The model under review builds one solid part; all positions refer to its coordinate system, in mm. Face numbers are marked on the shaded views. A direction names the side the tool comes from. Round coordinates to 2 decimals unless told otherwise and drop trailing zeros. Loops run counter-clockwise (first coordinate to the right, second up) from the corner with the lowest first, then second, coordinate; pieces in that order, holes last. Notation, with made-up numbers: (73, 62) -> (79, 62) arc R30 cw to (79, 101) -> close; hole circle Ø2 at (41, -18.75). An arc over 180 degrees is marked (long way). Write each question's results on one line, items separated by ' | '. Start each with the question number.
Item 1: Mouldability with a two-part tool opening along X and no side actions: class the marked faces 1, 2, 3 and 4 as pulls with the +X half, pulls with the -X half, needs draft (parallel to the pull), parting line crosses it, or undercut.
Item 2: Clearance check with flat-ended pins moving along their axes: pin 1 Ø2.5 at (y, z) = (0, 3) entering from -X; pin 2 Ø3.5 at (y, z) = (0, 3) entering from -X; pin 3 Ø2 at (x, z) = (-5.5, 4) entering from -Y; pin 4 Ø2 at (x, z) = (-7.5, 2) entering from -Y. State where each tip first meets the part, or that it passes through.
Item 3: We need section A-A (y = 0). Give the boundary of the cut face in (x, z).
Item 4: For L1, parallel to Z at x = -11.8, y = 0; L2, parallel to X at y = 6.5, z = 4.8; L3, parallel to Y at x = 0, z = 5.45, list the stretches that pass through material, from the lowest coordinate up. Write a range as from..to.
Item 5: Tool access review of the marked faces 5, 6 and 7: name each direction out of +Z, -Z, +X, -X, +Y, -Y from which nothing blocks a thin tool from reaching the whole face with its end or side.
Item 6: We need section C-C (x = 5). Give the boundary of the cut face in (y, z).
Item 7: We need section B-B (z = 0.4). Give the boundary of the cut face in (x, y).
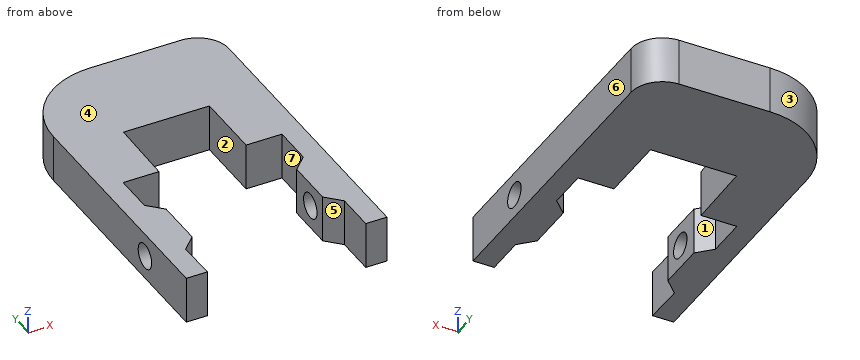
from build123d import *

# Parameters (mm, degrees)
PAD016_DEPTH    = 6
FILLET003_R     = 4
FILLET004_R     = 10
SKETCH047_R     = 1.6
POCKET022_DEPTH = 40


with BuildPart() as part:
    # Sketch046 → Pad016 (new body)
    with BuildSketch(Plane.XY):
        Polygon((10.115871, -9.866412), (10.115871, -4.766412), (8.315871, -2.966412), (8.315871, 3.233588), (10.115871, 5.033588), (10.115871, 10.133588), (5.545871, 10.133588), (5.545871, 18.880948), (-5.414129, 18.879181), (-5.564129, 10.133108), (-10.134129, 10.133108), (-10.134129, 5.033108), (-8.334129, 3.233108), (-8.334129, -2.966892), (-10.134129, -4.766892), (-10.064129, -9.866412), (-12.770461, -9.866412), (-12.770461, 31.817863), (12.822202, 31.817863), (12.822202, -9.866412), align=None)
    extrude(amount=PAD016_DEPTH)

    # Fillet003
    fillet003_edges = [part.edges().sort_by_distance(p)[0] for p in [
        (12.822202, 31.817863, 3),
    ]]
    fillet(fillet003_edges, radius=FILLET003_R)

    # Fillet004
    fillet004_edges = [part.edges().sort_by_distance(p)[0] for p in [
        (-12.770461, 31.817863, 3),
    ]]
    fillet(fillet004_edges, radius=FILLET004_R)

    # Sketch047 (on Face6 of Fillet004) → Pocket022 (cut)
    with BuildSketch(Plane(origin=(-12.770461, 0, 0), x_dir=(0, -1, 0), z_dir=(-1, 0, 0))):
        with Locations((0, 2.995476)):
            Circle(SKETCH047_R)
    extrude(amount=-POCKET022_DEPTH, mode=Mode.SUBTRACT)


solid = part.part
Here are the results:
1) face 1: undercut | face 2: undercut | face 3: pulls with the -X half | face 4: needs draft
2) pin 1: passes through | pin 2: stops at x = -12.77 | pin 3: stops at y = 10.13 | pin 4: stops at y = -3.13
3) outline: (-12.77, 0) -> (-8.33, 0) -> (-8.33, 1.4) -> (-12.77, 1.4) -> close; (-12.77, 4.6) -> (-8.33, 4.6) -> (-8.33, 6) -> (-12.77, 6) -> close; (8.32, 0) -> (12.82, 0) -> (12.82, 1.4) -> (8.32, 1.4) -> close; (8.32, 4.6) -> (12.82, 4.6) -> (12.82, 6) -> (8.32, 6) -> close
4) L1: z = 0..1.4, 4.6..6 | L2: x = -12.77..-10.13, 10.12..12.82 | L3: y = 18.88..31.82
5) face 5: +Z, -Z, -Y | face 6: +Z, -Z, +X, +Y, -Y | face 7: +Z, -Z
6) outline: (18.88, 0) -> (31.82, 0) -> (31.82, 6) -> (18.88, 6) -> close
7) outline: (-12.77, -9.87) -> (-10.06, -9.87) -> (-10.13, -4.77) -> (-8.33, -2.97) -> (-8.33, 3.23) -> (-10.13, 5.03) -> (-10.13, 10.13) -> (-5.56, 10.13) -> (-5.41, 18.88) -> (5.55, 18.88) -> (5.55, 10.13) -> (10.12, 10.13) -> (10.12, 5.03) -> (8.32, 3.23) -> (8.32, -2.97) -> (10.12, -4.77) -> (10.12, -9.87) -> (12.82, -9.87) -> (12.82, 27.82) arc R4 ccw to (8.82, 31.82) -> (-2.77, 31.82) arc R10 ccw to (-12.77, 21.82) -> close
